Input: part model. Units: mm. Frame: model coordinates. Face numbers are marked on the shaded views. Coordinates: 2 decimals unless noted, no trailing zeros. Order: outer loops, then holes, each group sorted by start corner. A loop starts at its lowest first (then second) coordinate and runs counter-clockwise, first axis right, second up. Notation, with made-up numbers: M 86.5,-9 L 137.5,-9 A25 ccw 137.5,21 Z; hole C 75.5,52 d9. An arc over 180 degrees is marked long. Answer in a Markdown table with one row per item.
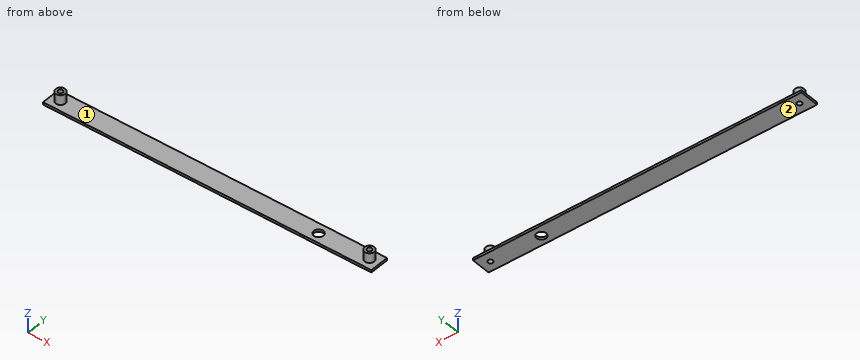
from build123d import *

# Parameters (mm, degrees)
SKETCH1_W           = 431.8
SKETCH1_H           = 25.4
SKETCH1_R           = 3.175
BOSS_EXTRUDE1_DEPTH = 3.175
SKETCH2_R           = 6.35
SKETCH2_R_2         = 3.175
BOSS_EXTRUDE2_DEPTH = 12.7
CUT_EXTRUDE1_REACH  = 5.175
SKETCH3_R           = 6.35


with BuildPart() as part:
    # Sketch1 → Boss-Extrude1 (new body)
    with BuildSketch(Plane.XY):
        with Locations((203.2, 0)):
            Rectangle(SKETCH1_W, SKETCH1_H)
        Circle(SKETCH1_R, mode=Mode.SUBTRACT)
        with Locations((406.4, 0)):
            Circle(SKETCH1_R, mode=Mode.SUBTRACT)
    extrude(amount=BOSS_EXTRUDE1_DEPTH)

    # Sketch2 → Boss-Extrude2 (add)
    with BuildSketch(Plane.XY.offset(3.175)):
        Circle(SKETCH2_R)
        Circle(SKETCH2_R_2, mode=Mode.SUBTRACT)
        with Locations((406.4, 0)):
            Circle(SKETCH2_R)
        with Locations((406.4, 0)):
            Circle(SKETCH2_R_2, mode=Mode.SUBTRACT)
    extrude(amount=BOSS_EXTRUDE2_DEPTH)

    # Sketch3 → Cut-Extrude1 (cut, up to next)
    with BuildSketch(Plane.XY.offset(3.175), mode=Mode.PRIVATE) as cut_extrude1_sk1:
        with Locations((339.668299959, -0.339967612)):
            Circle(SKETCH3_R)
    cut_extrude1_tool1 = extrude(cut_extrude1_sk1.sketch, amount=-CUT_EXTRUDE1_REACH, mode=Mode.PRIVATE) & part.part
    add(cut_extrude1_tool1.solids().sort_by_distance((339.6683, -0.339968, 3.175))[0], mode=Mode.SUBTRACT)


solid = part.part
1) Contact query for flat-ended pins moving along their axis: pin 1 (8 mm diameter, centred on x = 155, z = 11, fed in from +Y); pin 2 (5 mm diameter, centred on y = -9.5, z = 5, fed in from -X). Output: stop coordinate, or through.
Resolved:
| item | result |
|---|---|
| pin 1 | passes through |
| pin 2 | stops at x = -12.7 |
2) Cut plane A-A, the plane x = 233. Output: boundary loops of the cut face in (y, z) (3 decimals), and give its area (3 significant figures).
Resolved:
| item | result |
|---|---|
| outline | M -12.7,0 L 12.7,0 L 12.7,3.175 L -12.7,3.175 Z |
| area | 80.6 mm2 |
3) Material intervals for probe 1 along Y at (x, z) = (0, 5.75) (3 decimals); probe 2 along Z at (x, y) = (143, 1.75) (3 decimals); probe 3 along X at (y, z) = (-4.5, 12.5), sorted ascending.
Resolved:
| item | result |
|---|---|
| probe 1 | y = -6.35 to -3.175, 3.175 to 6.35 |
| probe 2 | z = 0 to 3.175 |
| probe 3 | x = -4.48 to 4.48, 401.92 to 410.88 |
4) Mould query, pull axis X, two halves, no side actions, for the marked faces 1 and 2. Classes: +X half, -X half, draft (parallel to the pull), parting line (faces both ways), or undercut.
Resolved:
| item | result |
|---|---|
| face 1 | undercut |
| face 2 | draft |
